Could you check a few things on this model? Use its own coordinates, in mm. Face numbers are marked on the shaded views. Round coordinates to 2 decimals unless told otherwise and drop trailing zeros. Order: outer loops, then holes, each group sorted by start corner. A loop starts at its lowest first (then second) coordinate and runs counter-clockwise, first axis right, second up. Notation, with made-up numbers: (28, 17.5) -> (79, 17.5) arc R20 cw to (79, 38.5) -> close; hole circle Ø9 at (23, -22.5). An arc over 180 degrees is marked (long way). Put each result on its own line as item: value. Start each with the question number.
Autodesk Inventor part; units mm, degrees
ref_plane "YZ Plane" through (0, 0, 0) normal (1, 0, 0) x (0, 1, 0)
ref_plane "XZ Plane" through (0, 0, 0) normal (0, 1, 0) x (-1, 0, 0)
ref_plane "XY Plane" through (0, 0, 0) normal (0, 0, 1) x (1, 0, 0)
sketch "Sketch1" plane through (0, 0, 0) normal (0, 1, 0) x (-1, 0, 0)
  line L0 (0, 0) -> (44.45, 0)
  line L1 (44.45, 0) -> (44.45, -10)
  line L2 (44.45, -10) -> (0, -10)
  line L3 (0, -10) -> (0, 0)
  dimension "d0" = 44.45
  dimension "d1" = 10
extrude "Extrusion1" add sketch "Sketch1" along normal blind 4
sketch "Sketch2" plane through (0, 4, 0) normal (0, 1, 0) x (1, 0, 0)
  circle A0 centre (-39.45, 5) radius 2.5
  circle A1 centre (-5, 5) radius 2.5
  line L0 (-44.45, 10) -> (-44.45, 0)
  point P0 (0, 0)
  dimension "d4" = 5
  dimension "d5" = 5
  dimension "d6" = 5
  dimension "d7" = 5
  dimension "d8" = 5
extrude "Extrusion2" cut sketch "Sketch2" against normal blind 8
fillet "Fillet1" radius 5 4 edges at (-44.45, 2, 0) (0, 2, 0) (0, 2, -10) (-44.45, 2, -10)
properties part number "Linkage" material "Aluminum 6061"
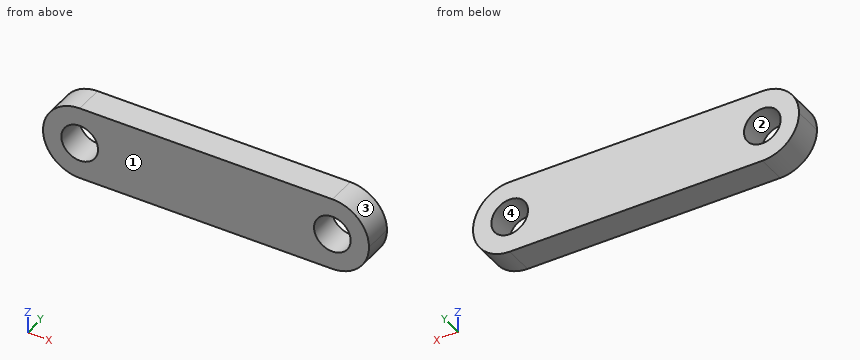
1. If we section it at D-D, the plane z = -1: Please give me the cut outline in (x, y), then the cut area to 3 significant figures.
2. Thinking about a two-plate mould opening in X: for the marked faces 1, 2, 3 and 4, which applies, +X half, -X half, draft (parallel to the pull), parting line (faces both ways), or undercut?
3. I need wall thicknesses on L1, parallel to X at y = 2.25, z = -5; L2, parallel to Z at x = -39.45, y = 2.95; L3, parallel to Z at x = -40.5, y = 1.75. Which ranges of each line are inside material? Lowest first, please.
4. If we section it at A-A, the plane y = 0.6: Count the separate pieces of the cut face and the enclosed holes in it, then the cut area to 3 significant figures.
5. If we section it at B-B, the plane z = -6: Please give me the cut outline in (x, y).
6. If we section it at C-C, the plane z = -3.5: Please give me the cut outline in (x, y).
Results below:
1. outline: (-42.45, 0) -> (-2, 0) -> (-2, 4) -> (-42.45, 4) -> close
1. area: 162 mm2
2. face 1: draft
2. face 2: undercut
2. face 3: +X half
2. face 4: undercut
3. L1: -44.45 to -41.95, -36.95 to -7.5, -2.5 to 0
3. L2: -10 to -7.5, -2.5 to 0
3. L3: -9.89 to -7.27, -2.73 to -0.11
4. separate pieces: 1
4. enclosed holes: 2
4. area: 384 mm2
5. outline: (-44.35, 0) -> (-41.74, 0) -> (-41.74, 4) -> (-44.35, 4) -> close; (-37.16, 0) -> (-7.29, 0) -> (-7.29, 4) -> (-37.16, 4) -> close; (-2.71, 0) -> (-0.1, 0) -> (-0.1, 4) -> (-2.71, 4) -> close
6. outline: (-44.22, 0) -> (-41.45, 0) -> (-41.45, 4) -> (-44.22, 4) -> close; (-37.45, 0) -> (-7, 0) -> (-7, 4) -> (-37.45, 4) -> close; (-3, 0) -> (-0.23, 0) -> (-0.23, 4) -> (-3, 4) -> close
